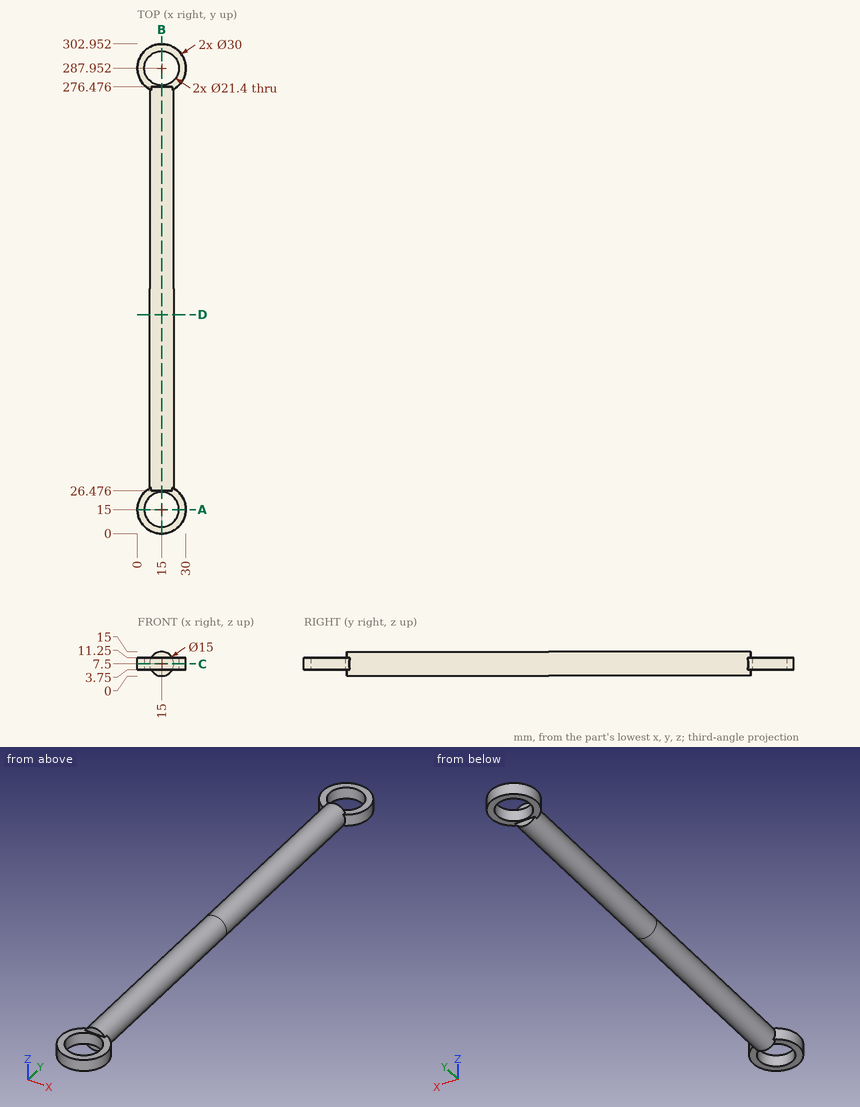
Could you check a few things on this drawing? It's one solid part, dimensions in mm from its lowest x, y, z. Give positions to 0.01 mm unless a question says otherwise; leave off trailing zeros. Loops run counter-clockwise (first coordinate to the right, second up) from the corner with the lowest first, then second, coordinate; pieces in that order, holes last. Notation, with made-up numbers: M 59,51.5 L 90,51.5 A18 ccw 90,57.5 Z; hole C -4.5,42 d7. An arc over 180 degrees is marked long. One line per question, with ' | ' between items. Start each with the question number.
Q1. If I drill on line 1 (Y direction, x = 16, z = 8.25) (1 decimal); line 2 (X direction, y = 14, z = 10.5); line 3 (Y direction, x = 8, z = 5.5) (1 decimal), over which ranges is the centre line in solid material (lowest first)? Write a range as from..to.
Q2. For pin 1 Ø17 at (x, y) = (15, 287.95) entering from +Z; pin 2 Ø1.9 at (x, z) = (16, 1.5) entering from -Y; pin 3 Ø1 at (x, y) = (11, 137) entering from -Z; pin 4 Ø8 at (y, z) = (84.5, 11) entering from -X, each with a flat end and sliding along its axis, tell me the tip position at first contact or that it passes through.
Q3. If we section it at C-C (z = 7.5): Please give me the cut outline in (x, y), plus the area to 3 significant figures.
Q4. If we section it at B-B (x = 15): Please give me the cut outline in (y, z).
Q5. If we section it at A-A (y = 15): Please give me the cut outline in (x, z), plus the area to 3 significant figures.
Q6. If we section it at D-D (y = 135.5): Please give me the cut outline in (x, z), plus the area to 3 significant figures.
Computed:
1) line 1: y = 0..4.3, 25.7..277.3, 298.6..302.9 | line 2: x = 0.03..4.35, 25.65..29.97 | line 3: y = 1.7..6.9, 23.1..279.9, 296..301.2
2) pin 1: passes through | pin 2: stops at y = 26.48 | pin 3: stops at z = 0.87 | pin 4: stops at x = 7.5
3) outline: M 7.5,27.99 A15 ccw long 22.5,27.99 L 22.5,274.96 A15 ccw long 7.5,274.96 Z; hole C 15,15 d21.4; hole C 15,287.95 d21.4 | area: 4,360 mm²
4) outline: M 0,3.75 L 4.3,3.75 L 4.3,11.25 L 0,11.25 Z; M 25.7,3.75 L 26.48,3.75 L 26.48,0 L 276.48,0 L 276.48,3.75 L 277.25,3.75 L 277.25,11.25 L 276.48,11.25 L 276.48,15 L 26.48,15 L 26.48,11.25 L 25.7,11.25 Z; M 298.65,3.75 L 302.95,3.75 L 302.95,11.25 L 298.65,11.25 Z
5) outline: M 0,3.75 L 4.3,3.75 L 4.3,11.25 L 0,11.25 Z; M 25.7,3.75 L 30,3.75 L 30,11.25 L 25.7,11.25 Z | area: 64.5 mm²
6) outline: C 15,7.5 d15 | area: 177 mm²
